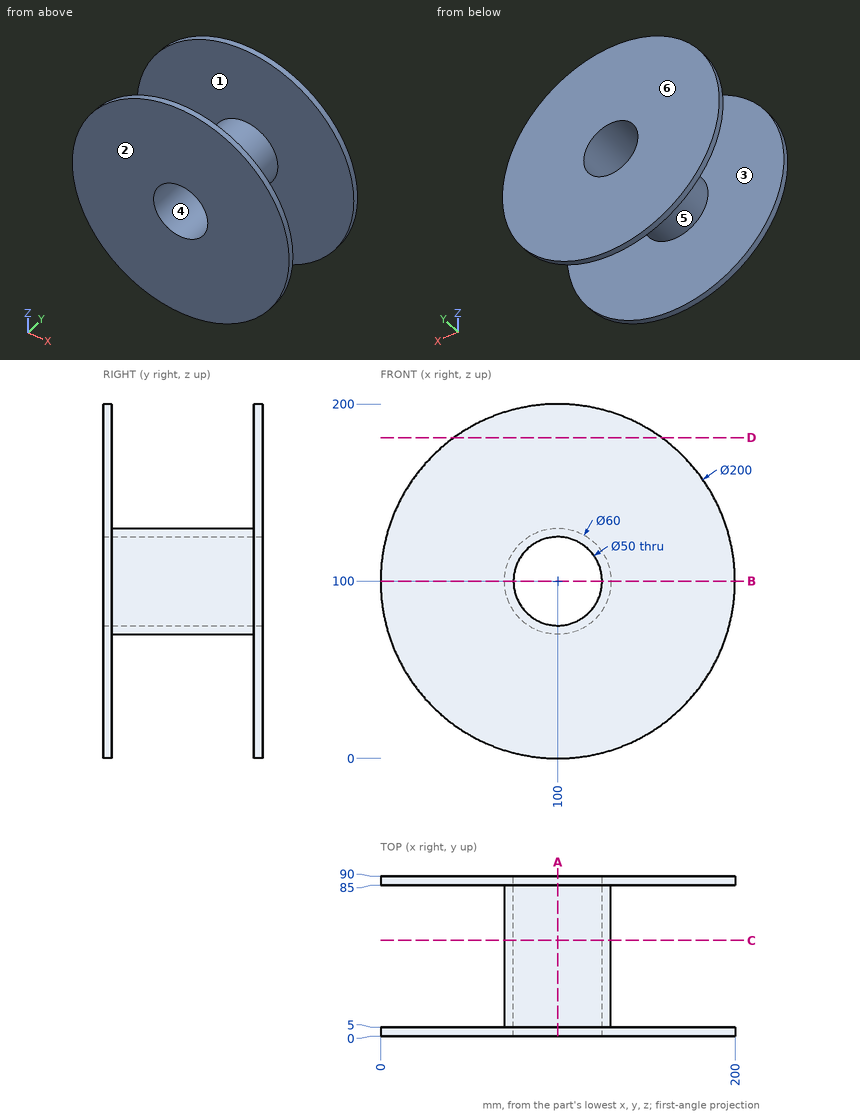
Study the drawing (mm; zero at the part's minimum x, y, z) and answer. A direction names the side the tool comes from. Round coordinates to 2 decimals unless told otherwise and drop trailing zeros. Loops run counter-clockwise (first coordinate to the right, second up) from the corner with the lowest first, then second, coordinate; pieces in that order, holes last. Notation, with made-up numbers: (62, 25) -> (96, 25) arc R27 ccw to (96, 50) -> close; hole circle Ø8 at (50.25, -12.5). An arc over 180 degrees is marked (long way). Write each question's results on one line, items separated by ' | '. Start each with the question number.
1. Section C-C (y = 54) is taken. Determine the outline of the cut face in (x, z), plus the area to 3 significant figures.
2. Section B-B (z = 100) is taken. Determine the outline of the cut face in (x, y), plus the area to 3 significant figures.
3. A tool of negligible diameter and unlimited length cuts with its end or side. For the marked faces 5 and 6, from which of +Z, -Z, +X, -X, +Y, -Y can it reach the whole face along a straight path? Write none if from no direction.
4. Given pin 1 Ø2 at (x, z) = (20, 164.5) entering from +Y; pin 2 Ø1.5 at (x, z) = (109, 138) entering from -Y, each flat-ended and moving along its own axis, determine where each tip first touches the part or whether it passes through.
5. For a pull along Y with two mould halves and no side action, classify the marked faces 1, 2, 3 and 4 as +Y half, -Y half, draft (parallel to the pull), parting line (faces both ways), or undercut.
6. Section D-D (z = 181) is taken. Determine the outline of the cut face in (x, y).
7. Find the intervals of material crossed by probe 1 along Y at (x, z) = (77, 177); probe 2 along Z at (x, y) = (100, 60); probe 3 along X at (y, z) = (53.5, 99), in increasing order. Write a range as from..to.
8. Section A-A (x = 100) is taken. Determine the outline of the cut face in (y, z), plus the area to 3 significant figures.
Evaluation:
1) outline: circle Ø60 at (100, 100); hole circle Ø50 at (100, 100) | area: 864 mm2
2) outline: (0, 0) -> (75, 0) -> (75, 90) -> (0, 90) -> (0, 85) -> (70, 85) -> (70, 5) -> (0, 5) -> close; (125, 0) -> (200, 0) -> (200, 5) -> (130, 5) -> (130, 85) -> (200, 85) -> (200, 90) -> (125, 90) -> close | area: 2,300 mm2
3) face 5: none | face 6: +Z, -Z, +X, -X, +Y
4) pin 1: passes through | pin 2: stops at y = 0
5) face 1: undercut | face 2: -Y half | face 3: undercut | face 4: draft
6) outline: (41.36, 0) -> (158.64, 0) -> (158.64, 5) -> (41.36, 5) -> close; (41.36, 85) -> (158.64, 85) -> (158.64, 90) -> (41.36, 90) -> close
7) probe 1: y = 0..5, 85..90 | probe 2: z = 70..75, 125..130 | probe 3: x = 70.02..75.02, 124.98..129.98
8) outline: (0, 0) -> (5, 0) -> (5, 70) -> (85, 70) -> (85, 0) -> (90, 0) -> (90, 75) -> (0, 75) -> close; (0, 125) -> (90, 125) -> (90, 200) -> (85, 200) -> (85, 130) -> (5, 130) -> (5, 200) -> (0, 200) -> close | area: 2,300 mm2
